Can you work these out from the model? Positions are in its coordinate system, mm. Face numbers are marked on the shaded views. Give positions to 0.01 mm unless a question says otherwise; leave off trailing zeros. Write each loop counter-clockwise with the first axis right and the second up, starting at its lowest first coordinate (ties: lowest second). Pieces come first, ordered by that corner, then holes.
1. Suppose I cut it at B-B (x = 0). Please give me the cut outline in (y, z).
2. Suppose I cut it at A-A (z = 34.5). Please give me the cut outline in (x, y), and give its area (3 significant figures).
3. If I drill on probe 1 along Y at (x, z) = (26.5, 58); probe 2 along X at (y, z) = (-35, 26); probe 3 along Z at (x, y) = (0, -18), over which ranges is the centre line in solid material (lowest first)?
4. I'm going to push flat-ended pins straight in: pin 1 (8 mm diameter, centred on x = 15.5, z = 29, fed in from +Y); pin 2 (12 mm diameter, centred on x = 17, y = -29, fed in from +Z); pin 3 (3 mm diameter, centred on x = 34, z = 147.5, fed in from -Y); pin 4 (12 mm diameter, centred on x = 17.5, y = -20, fed in from +Z). Where does each tip first touch, or does it pass through?
5. Suppose I cut it at D-D (z = 177.5). Please give me the cut outline in (x, y).
6. Thinking about a two-plate mould opening in X: for the marked faces 1, 2 and 3, which applies, pulls with the +X half, pulls with the -X half, needs draft (parallel to the pull), parting line crosses it, or undercut?
7. Suppose I cut it at C-C (y = -24). Please give me the cut outline in (x, z), and give its area (3 significant figures).
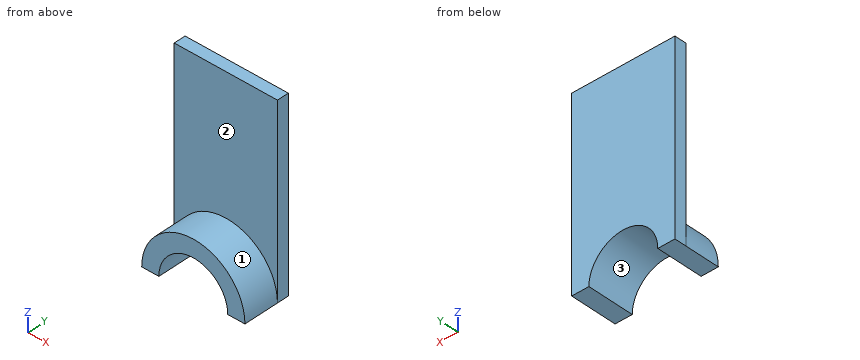
```python
from build123d import *

# Parameters (mm, degrees)
F1_W     = 112.0290251324
F1_H     = 201.4646567404
F2_DEPTH = 12.7
F3_DEPTH = 50.8
F4_DEPTH = 25.4


with BuildPart() as f2:
    # F1 (on Front) → F2 (new body)
    with BuildSketch(Plane.XZ):
        with Locations((0, 100.7323283702)):
            Rectangle(F1_W, F1_H)
    extrude(amount=F2_DEPTH)

    # F0 (on Front) → F3 (join)
    with BuildSketch(Plane.XZ):
        with BuildLine():
            ThreePointArc((-37.3730720306, 0), (0, 37.3730720306), (37.3730720306, 0))
            Line((37.3730720306, 0), (56.0145125662, 0))
            ThreePointArc((56.0145125662, 0), (0, 56.0145125662), (-56.0145125662, 0))
            Line((-56.0145125662, 0), (-37.3730720306, 0))
        make_face()
    extrude(amount=F3_DEPTH)

    # F4 (cut): a face of the model
    f4_faces = [f2.faces().sort_by_distance(p)[0] for p in [
        (0, -12.7, 15.8616244059),
    ]]
    extrude(f4_faces, amount=-F4_DEPTH, mode=Mode.SUBTRACT)


solid = f2.part
```
Checks:
1. outline: (-50.8, 37.37) - (0, 37.37) - (0, 201.46) - (-12.7, 201.46) - (-12.7, 56.01) - (-50.8, 56.01) - close
2. outline: (-56.01, -12.7) - (-44.13, -12.7) - (-44.13, -50.8) - (-14.37, -50.8) - (-14.37, 0) - (-56.01, 0) - close; (14.37, -50.8) - (44.13, -50.8) - (44.13, -12.7) - (56.01, -12.7) - (56.01, 0) - (14.37, 0) - close
2. area: 3,330 mm2
3. probe 1: y = -12.7 to 0
3. probe 2: x = -49.61 to -26.85, 26.85 to 49.61
3. probe 3: z = 37.37 to 56.01
4. pin 1: passes through
4. pin 2: stops at z = 54.92
4. pin 3: stops at y = -12.7
4. pin 4: stops at z = 54.82
5. outline: (-56.01, -12.7) - (56.01, -12.7) - (56.01, 0) - (-56.01, 0) - close
6. face 1: parting line crosses it
6. face 2: needs draft
6. face 3: undercut
7. outline: (-56.01, 0) - (-37.37, 0) arc R37.37 cw to (37.37, 0) - (56.01, 0) arc R56.01 ccw to start
7. area: 2,730 mm2
